from build123d import *

# Parameters (mm, degrees)
SKETCH2_W           = 635
SKETCH2_H           = 635
BOSS_EXTRUDE3_DEPTH = 4.445
SKETCH3_R           = 3.175
SKETCH3_R_2         = 3.9751
CUT_EXTRUDE1_DEPTH  = 514.410627343
SKETCH5_W           = 635
SKETCH5_H           = 635
CUT_EXTRUDE2_DEPTH  = 514.410627343
CUT_EXTRUDE3_DEPTH  = 359.355916807
SKETCH10_R          = 3.175
CUT_EXTRUDE5_DEPTH  = 359.355916807


with BuildPart() as part:
    # Sketch2 → Boss-Extrude3 (new body)
    with BuildSketch(Plane.XY):
        with Locations((84.381748098, -1.971086)):
            Rectangle(SKETCH2_W, SKETCH2_H)
    extrude(amount=BOSS_EXTRUDE3_DEPTH)

    # Sketch3 → Cut-Extrude1 (cut, through all)
    with BuildSketch(Plane(origin=(0, 0, 0), x_dir=(-1, 0, 0), z_dir=(0, 0, -1))):
        with Locations((-130.02651813, 72.45351862)):
            Circle(SKETCH3_R)
        with Locations((-195.288059763, -21.383687133)):
            Circle(SKETCH3_R)
        with Locations((-122.004659563, -96.265887155)):
            Circle(SKETCH3_R)
        with Locations((-26.754659563, -96.265887155)):
            Circle(SKETCH3_R)
        with Locations((-26.754659563, 23.469712845)):
            Circle(SKETCH3_R_2)
        with Locations((81.195340437, -96.265887155)):
            Circle(SKETCH3_R)
        with Locations((-299.804659563, -96.265887155)):
            Circle(SKETCH3_R)
        with Locations((81.195340437, 23.469712845)):
            Circle(SKETCH3_R)
        with Locations((-299.804659563, 23.469712845)):
            Circle(SKETCH3_R)
    extrude(amount=-CUT_EXTRUDE1_DEPTH, mode=Mode.SUBTRACT)

    # Sketch5 → Cut-Extrude2 (cut, through all)
    with BuildSketch(Plane.XY.offset(4.445)):
        with Locations((84.381748098, -1.971086)):
            Rectangle(SKETCH5_W, SKETCH5_H)
        Polygon((-106.595340437, -121.665887155), (325.204659563, -121.665887155), (325.204659563, 48.869712845), (141.054659563, 150.469712845), (77.554659563, 150.469712845), (-106.595340437, 48.869712845), align=None, mode=Mode.SUBTRACT)
    extrude(amount=-CUT_EXTRUDE2_DEPTH, mode=Mode.SUBTRACT)

    # Sketch7 → Cut-Extrude3 (cut, through all)
    with BuildSketch(Plane.XY.offset(4.445)):
        with BuildLine():
            ThreePointArc((-106.595340437, -96.265887155), (-96.435340437, -36.398087155), (-106.595340437, 23.469712845))
            Line((-106.595340437, 23.469712845), (-106.595340437, -96.265887155))
        make_face()
        with BuildLine():
            ThreePointArc((299.804659563, -121.665887155), (109.304659563, -111.505887155), (-81.195340437, -121.665887155))
            Line((-81.195340437, -121.665887155), (299.804659563, -121.665887155))
        make_face()
        with BuildLine():
            ThreePointArc((325.204659563, 23.469712845), (315.044659563, -36.398087155), (325.204659563, -96.265887155))
            Line((325.204659563, -96.265887155), (325.204659563, 23.469712845))
        make_face()
        with BuildLine():
            Line((55.314986389, 138.199548335), (-84.355667262, 61.139877355))
            ThreePointArc((-84.355667262, 61.139877355), (-9.612274633, 90.773843575), (55.314986389, 138.199548335))
        make_face()
        with BuildLine():
            Line((302.964986389, 61.139877355), (163.294332738, 138.199548335))
            ThreePointArc((163.294332738, 138.199548335), (228.221593759, 90.773843575), (302.964986389, 61.139877355))
        make_face()
    extrude(amount=-CUT_EXTRUDE3_DEPTH, mode=Mode.SUBTRACT)

    # Sketch10 → Cut-Extrude5 (cut, through all)
    with BuildSketch(Plane.XY.offset(4.445)):
        with Locations((109.304659563, 131.419712845)):
            Circle(SKETCH10_R)
        with Locations((109.304659563, 99.669712845)):
            Circle(SKETCH10_R)
    extrude(amount=-CUT_EXTRUDE5_DEPTH, mode=Mode.SUBTRACT)


solid = part.part
Work out the finished part from the listing and answer in its coordinate system (mm). Give positions to 0.01 mm unless a question says otherwise; leave off trailing zeros. Write each loop counter-clockwise with the first axis right and the second up, starting at its lowest first coordinate (ties: lowest second). Pieces come first, ordered by that corner, then holes.
Q1. Straight lines are drawn through the part: L1, parallel to Y at x = 122, z = 2.95; L2, parallel to Y at x = 107, z = 2.15; L3, parallel to X at y = 132.5, z = 2.8. For each, find the intervals that lie inside material, in ascending order.
Answer:
L1: y = -111.55 to -99.44, -93.09 to 150.47
L2: y = -111.51 to 97.49, 101.85 to 129.24, 133.6 to 150.47
L3: x = 49.13 to 106.32, 112.29 to 169.48
Q2. Given pin 1 (1.5 mm diameter, centred on y = -39.5, z = 1.5, fed in from +X); pin 2 (1 mm diameter, centred on y = -53, z = 2.5, fed in from -X); pin 3 (2 mm diameter, centred on x = 34, z = 4, fed in from +Y), each flat-ended and moving along its own axis, determine where each tip first touches the part or whether it passes through.
Answer:
pin 1: stops at x = 315.09
pin 2: stops at x = -97.24
pin 3: stops at y = 120.55
Q3. The part is cut by section A-A on z = 3.4. State how many separate pieces and enclosed holes the cut face has, and give its area (3 significant figures).
Answer:
separate pieces: 1
enclosed holes: 11
area: 92,100 mm2
Q4. The part is cut by section B-B on y = 9. Give the vertices of the cut face in (x, z) (3 decimals).
Answer:
outline: (-102.206, 0) - (320.815, 0) - (320.815, 4.445) - (-102.206, 4.445) - close
Q5. The part is cut by section C-C on x = -11. Give the vertices of the cut face in (y, z) (3 decimals), and give its area (3 significant figures).
Answer:
outline: (-115.551, 0) - (90.013, 0) - (90.013, 4.445) - (-115.551, 4.445) - close
area: 914 mm2
Q6. For a pull along X with two mould halves and no side action, classify faces 1 (the face through (111.977, -111.508, 2.254)), 2 (the face through (106, -14, 4.445)), 3 (the face through (-96.437, -37.252, 2.254)) as released by +X, released by -X, zero draft, split by the parting line, or undercut.
Answer:
face 1: undercut
face 2: zero draft
face 3: released by -X
